Design review of the part built by this model. Coordinates are the model's own, in mm. Face numbers are marked on the shaded views. Coordinates: 2 decimals unless noted, no trailing zeros. Loops run counter-clockwise (first coordinate to the right, second up) from the corner with the lowest first, then second, coordinate; pieces in that order, holes last. Notation, with made-up numbers: (-35, 6.5) -> (-16, 6.5) arc R26 ccw to (-16, 31.5) -> close; hole circle Ø6 at (-5.75, 75.5). An arc over 180 degrees is marked (long way). One line per item, written item: value. Start each with the question number.
1. Add section A-A on y = 0. Write out the cut boundary in (x, z).
2. Draft analysis for pull direction Y (two halves, no side actions). For the marked faces 1, 2 and 3, state which applies: pulls with the +Y half, pulls with the -Y half, needs draft (parallel to the pull), parting line crosses it, or undercut.
3. Add section C-C on z = 2.65. Write out the cut boundary in (x, y), plus the area to 3 significant figures.
4. Insertion check: pin 1 (2 mm diameter, centred on x = 2.5, z = 5, fed in from -Y); pin 2 (1 mm diameter, centred on y = -2, z = 4, fed in from +X). Each pin has a flat end and moves straight along its axis. Give the tip position at first contact, or say it passes through.
5. For probe 1 along X at (y, z) = (0, 2.7); probe 2 along Y at (x, z) = (-0.5, 3.75), list the stretches that pass through material, from the lowest coordinate up.
6. Add section D-D on z = 3.5. Write out the cut boundary in (x, y).
```python
from build123d import *

# Parameters (mm, degrees)
F0_R        = 6
F0_R_2      = 4
F0_R_3      = 1.75
F1_DEPTH    = 6
F2_R        = 1
F3_SIZE     = 3
F1_FACE_R   = 6
F1_FACE_R_2 = 1.75
F4_DEPTH    = 2.28


with BuildPart() as f1:
    # F0 (on Top) → F1 (new body)
    with BuildSketch(Plane.XY):
        Circle(F0_R)
        Circle(F0_R_2, mode=Mode.SUBTRACT)
        Circle(F0_R_2)
        Circle(F0_R_3, mode=Mode.SUBTRACT)
    extrude(amount=F1_DEPTH)

    # F2
    f2_edges = [f1.edges().sort_by_distance(p)[0] for p in [
        (-6, 0, 6),
    ]]
    fillet(f2_edges, radius=F2_R)

    # F3
    f3_edges = [f1.edges().sort_by_distance(p)[0] for p in [
        (-1.75, 0, 6),
    ]]
    chamfer(f3_edges, length=F3_SIZE)

    # F1_face (on face) → F4 (cut)
    with BuildSketch(Plane(origin=(0, 0, 0), x_dir=(1, 0, 0), z_dir=(0, 0, -1))):
        Circle(F1_FACE_R)
        Circle(F1_FACE_R_2, mode=Mode.SUBTRACT)
    extrude(amount=-F4_DEPTH, mode=Mode.SUBTRACT)


solid = f1.part
```
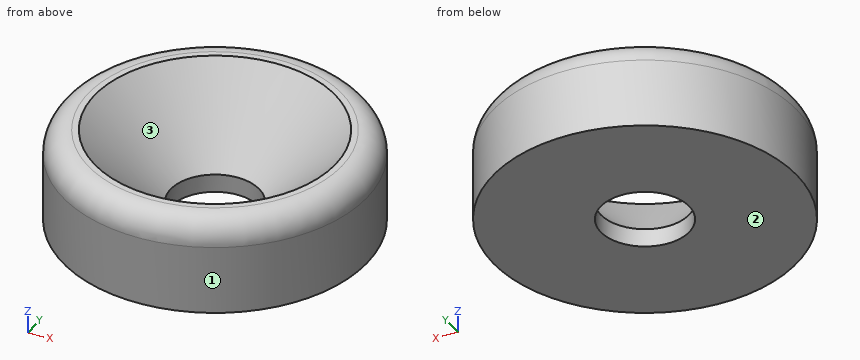
Worked answers:
1. outline: (-6, 2.28) -> (-1.75, 2.28) -> (-1.75, 3) -> (-4.75, 6) -> (-5, 6) arc R1 ccw to (-6, 5) -> close; (1.75, 2.28) -> (6, 2.28) -> (6, 5) arc R1 ccw to (5, 6) -> (4.75, 6) -> (1.75, 3) -> close
2. face 1: parting line crosses it
2. face 2: needs draft
2. face 3: undercut
3. outline: circle Ø12 at (0, 0); hole circle Ø3.5 at (0, 0)
3. area: 103 mm²
4. pin 1: stops at y = -5.81
4. pin 2: stops at x = 5.81
5. probe 1: x = -6 to -1.75, 1.75 to 6
5. probe 2: y = -5.98 to -2.45, 2.45 to 5.98
6. outline: circle Ø12 at (0, 0); hole circle Ø4.5 at (0, 0)
